Could you check a few things on this model? Use its own coordinates, in mm. Face numbers are marked on the shaded views. A direction names the side the tool comes from. Give positions to 0.01 mm unless a question says otherwise; leave off trailing zeros. Order: outer loops, then holes, each group sorted by start corner. A loop starts at its lowest first (then second) coordinate and runs counter-clockwise, first axis right, second up. Notation, with made-up numbers: M 64,46.25 L 116,46.25 A24 ccw 116,71.25 Z; hole C 61.25,27 d6. An arc over 180 degrees is marked long. Answer in a Markdown table with one row per item. Add a question column.
Autodesk Inventor part; units mm, degrees
ref_plane "YZ Plane" through (0, 0, 0) normal (1, 0, 0) x (0, 1, 0)
ref_plane "XZ Plane" through (0, 0, 0) normal (0, 1, 0) x (-1, 0, 0)
ref_plane "XY Plane" through (0, 0, 0) normal (0, 0, 1) x (1, 0, 0)
sketch "Sketch1" plane through (0, 0, 0) normal (0, 0, 1) x (1, 0, 0)
  line L0 (57.5, 0) -> (28.75, -49.7965)
  line L1 (28.75, -49.7965) -> (-28.75, -49.7965)
  line L2 (-28.75, -49.7965) -> (-57.5, 0)
  line L3 (-57.5, 0) -> (-28.75, 49.7965)
  line L4 (-28.75, 49.7965) -> (28.75, 49.7965)
  line L5 (28.75, 49.7965) -> (57.5, 0)
  point P0 (0, 0)
  point P1 (0, 0)
  dimension "d0" = 115
extrude "Extrusion1" add sketch "Sketch1" along normal blind 40
sketch "Sketch2" plane through (0, 0, 0) normal (0, 0, -1) x (-1, 0, 0)
  line L0 (-73, 53) -> (73, 53)
  line L1 (73, 53) -> (73, -53)
  line L2 (73, -53) -> (-73, -53)
  line L3 (-73, -53) -> (-73, 53)
  point P0 (0, 0)
  point P1 (0, 53)
  point P2 (-73, 0)
  dimension "d3" = 146
  dimension "d4" = 106
extrude "Extrusion2" add sketch "Sketch2" along normal blind 105
sketch "Sketch3" plane through (0, 0, 40) normal (0, 0, 1) x (1, 0, 0)
  circle A0 centre (0, 0) radius 25
  dimension "d7" = 50
extrude "Extrusion3" cut sketch "Sketch3" against normal blind 5
sketch "Sketch4" plane through (0, 0, -105) normal (0, 0, -1) x (-1, 0, 0)
  line L0 (56, 11.5) -> (-56, 11.5)
  line L1 (-56, 11.5) -> (-56, -11.5)
  line L2 (-56, -11.5) -> (56, -11.5)
  line L3 (56, -11.5) -> (56, 11.5)
  point P0 (0, 0)
  point P1 (56, 0)
  point P2 (0, 11.5)
  dimension "d10" = 23
  dimension "d11" = 112
extrude "Extrusion4" cut sketch "Sketch4" against normal blind 20
properties part number "link_g0" material "ABS Plastic"
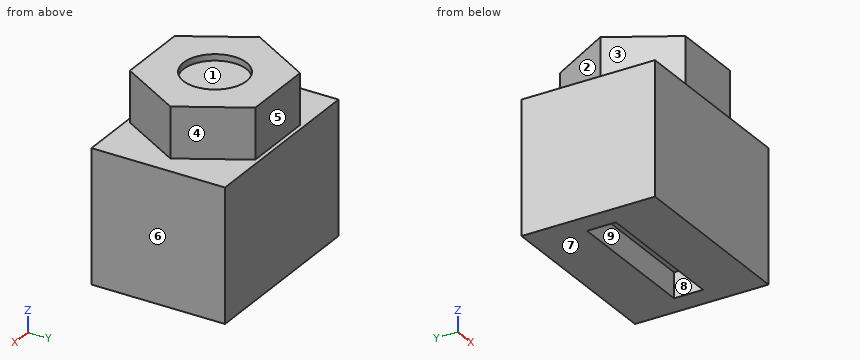
1. For the marked faces 1, 2, 3, 4 and 5, which set-ups out of +Z, -Z, +X, -X, +Y, -Y let a thin tool reach every point of the face, with its end or its side?
2. If I drill on line 1 along Y through (x, z) = (0, 37.65); line 2 along Z through (x, y) = (11.5, 8); line 3 along Z through (x, y) = (48.5, 32), over which ranges is the centre line in solid material (lowest first)? Write a range as [from, to].
3. Suppose I cut it at C-C on z = 2.5. List the corners of the cut face in (x, y) for me.
4. Suppose I cut it at D-D on y = -16. List the corners of the cut face in (x, z) for me, plus the area to 3 significant figures.
5. Suppose I cut it at A-A on x = 0. List the corners of the cut face in (y, z) for me, plus the area to 3 significant figures.
6. Suppose I cut it at B-B on y = 46.5. List the corners of the cut face in (x, z) for me.
7. Thinking about a two-plate mould opening in X: for the marked faces 6, 7, 8 and 9, which applies, pulls with the +X half, pulls with the -X half, needs draft (parallel to the pull), parting line crosses it, or undercut?
8. Will these pins go through, and if not, where does the flat tip stop? P1, Ø18.5, axis at x = 16.5, y = -1.5, coming from the -Z side; P2, Ø1, axis at y = -12, z = 19, coming from the -X side; P3, Ø15, axis at x = 9, y = -8, coming from the +Z side.
Findings below:
| question | item | result |
|---|---|---|
| 1 | face 1 | +Z |
| 1 | face 2 | +Z, -X, +Y |
| 1 | face 3 | +Z, -X, -Y |
| 1 | face 4 | +Z, +X, +Y |
| 1 | face 5 | +Z, +X, -X, +Y |
| 2 | line 1 | [-49.8, -25], [25, 49.8] |
| 2 | line 2 | [-85, 35] |
| 2 | line 3 | [-105, 0] |
| 3 | outline | M -57.5,0 L -28.75,-49.8 L 28.75,-49.8 L 57.5,0 L 28.75,49.8 L -28.75,49.8 Z |
| 4 | outline | M -73,-105 L 73,-105 L 73,0 L 48.26,0 L 48.26,40 L 19.21,40 L 19.21,35 L -19.21,35 L -19.21,40 L -48.26,40 L -48.26,0 L -73,0 Z |
| 4 | area | 19,000 mm2 |
| 5 | outline | M -53,-105 L -11.5,-105 L -11.5,-85 L 11.5,-85 L 11.5,-105 L 53,-105 L 53,0 L 49.8,0 L 49.8,40 L 25,40 L 25,35 L -25,35 L -25,40 L -49.8,40 L -49.8,0 L -53,0 Z |
| 5 | area | 14,400 mm2 |
| 6 | outline | M -73,-105 L 73,-105 L 73,0 L 30.65,0 L 30.65,40 L -30.65,40 L -30.65,0 L -73,0 Z |
| 7 | face 6 | pulls with the +X half |
| 7 | face 7 | needs draft |
| 7 | face 8 | undercut |
| 7 | face 9 | undercut |
| 8 | P1 | z = -85 |
| 8 | P2 | x = -50.86 |
| 8 | P3 | z = 35 |
